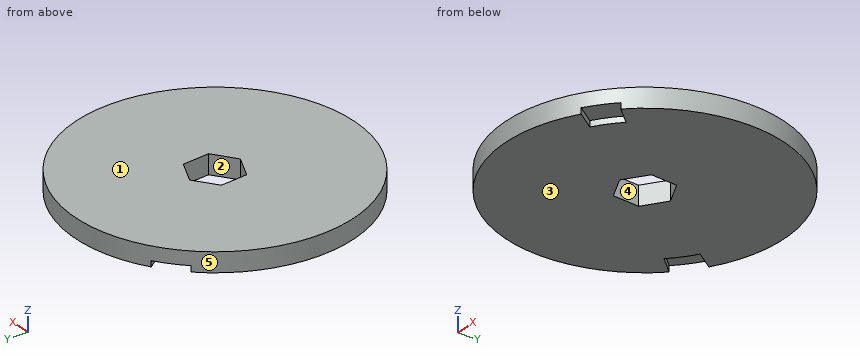
from build123d import *

# Parameters (mm, degrees)
SKETCH_1_R               = 35.9
EXTRUDE_1_DEPTH          = 5
CUT_EXTRUDE_1_DEPTH      = 1.5
PATTERN_CIRCULAR_1_COUNT = 2


with BuildPart() as part:
    # 草图1 → 凸台-拉伸1 (new body)
    with BuildSketch(Plane.XY):
        Circle(SKETCH_1_R)
        Polygon((6.292659869, -3.066338496), (5.801856968, 3.916434056), (-0.490802901, 6.982772552), (-6.292659869, 3.066338496), (-5.801856968, -3.916434056), (0.490802901, -6.982772552), align=None, mode=Mode.SUBTRACT)
    extrude(amount=EXTRUDE_1_DEPTH)

    # 草图2 → 切除-拉伸1 (cut)
    with BuildSketch(Plane(origin=(0, 0, 0), x_dir=(-1, 0, 0), z_dir=(0, 0, -1))):
        with BuildLine():
            Line((18.682261423, 30.655882113), (15.242196262, 25.839416656))
            ThreePointArc((15.242196262, 25.839416656), (18.484517825, 23.628851025), (21.410564164, 21.013989202))
            Line((21.410564164, 21.013989202), (25.403819071, 25.366434054))
            ThreePointArc((25.403819071, 25.366434054), (22.201130343, 28.21205082), (18.682261423, 30.655882113))
        make_face()
    cut_extrude_1 = extrude(amount=-CUT_EXTRUDE_1_DEPTH, mode=Mode.SUBTRACT)

    # 阵列(圆周)1: 切除-拉伸1 ×2 about axis
    pattern_circular_1_axis = Axis((0, 0, 0), (0, 0, 1))
    for i in range(1, PATTERN_CIRCULAR_1_COUNT):
        add(cut_extrude_1.rotate(pattern_circular_1_axis, i * 360 / PATTERN_CIRCULAR_1_COUNT), mode=Mode.SUBTRACT)


solid = part.part
Input: part model. Units: mm. Frame: model coordinates. Face numbers are marked on the shaded views. A direction names the side the tool comes from. Coordinates: 2 decimals unless noted, no trailing zeros. Loops run counter-clockwise (first coordinate to the right, second up) from the corner with the lowest first, then second, coordinate; pieces in that order, holes last. Notation, with made-up numbers: (12, -15.75) -> (33, -15.75) arc R5 ccw to (33, -10.75) -> close; hole circle Ø9 at (65.25, 61). An arc over 180 degrees is marked (long way). Write each question's results on one line, items separated by ' | '. Start each with the question number.
Q1. Ray query, line 1 (X direction, y = -2, z = 4.7); line 2 (X direction, y = -5.5, z = 2.4); line 3 (Y direction, x = -2.5, z = 0.75). Return the intervals inside material, ascending. Write a range as from..to.
Q2. Section C-C, the plane x = -12.5. Return the cut outline in (y, z), plus the area to 3 significant figures.
Q3. Section D-D, the plane y = 19. Return the cut outline in (x, z), plus the area to 3 significant figures.
Q4. Pull-direction query (X, two-part tool) for the marked faces 3, 4 and 5; classes: released by +X, released by -X, zero draft, split by the parting line, or undercut.
Q5. Section B-B, the plane y = 0. Return the cut outline in (x, z).
Q6. Reachability of the marked faces 1 and 2 from +Z, -Z, +X, -X, +Y, -Y: full face, straight path, thin tool, end or side. Return the list, or none.
Q7. Section A-A, the plane z = 2.9. Return the cut outline in (x, y), plus the area to 3 significant figures.
Q8. Pin query (flat end, axial travel): pin 1 (2 mm diameter, centred on x = -7, z = 1, fed in from +Y); pin 2 (1 mm diameter, centred on x = -15, z = 2, fed in from -Y). Return the tip coordinate at first contact, or that it passes through.
Found:
1) line 1: -35.84..-5.94, 6.22..35.84 | line 2: -35.48..-2.55, 2.69..35.48 | line 3: -35.81..-5.53, 5.63..35.81
2) outline: (-33.65, 0) -> (33.65, 0) -> (33.65, 5) -> (-33.65, 5) -> close | area: 337 mm2
3) outline: (-30.46, 0) -> (30.46, 0) -> (30.46, 5) -> (-30.46, 5) -> close | area: 305 mm2
4) face 3: zero draft | face 4: undercut | face 5: split by the parting line
5) outline: (-35.9, 0) -> (-6.08, 0) -> (-6.08, 5) -> (-35.9, 5) -> close; (6.08, 0) -> (35.9, 0) -> (35.9, 5) -> (6.08, 5) -> close
6) face 1: +Z, +X, -X, +Y, -Y | face 2: +Z, -Z
7) outline: circle Ø71.8 at (0, 0); hole (-6.29, 3.07) -> (-5.8, -3.92) -> (0.49, -6.98) -> (6.29, -3.07) -> (5.8, 3.92) -> (-0.49, 6.98) -> close | area: 3,920 mm2
8) pin 1: y = 35.4 | pin 2: y = -32.84
